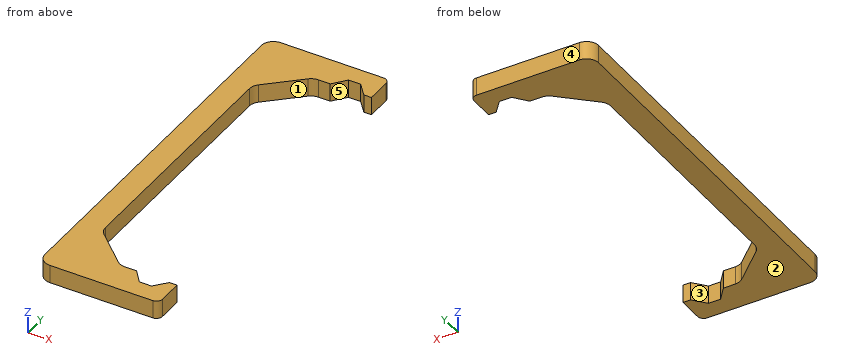
```python
from build123d import *

# Parameters (mm, degrees)
F1_DEPTH = 9.525


with BuildPart() as f1:
    # F0 (on Top) → F1 (new body)
    with BuildSketch(Plane.XY):
        with BuildLine():
            Line((-2.285999, 147.979229), (-46.735999, 147.979229))
            ThreePointArc((-46.735999, 147.979229), (-51.226127, 146.119357), (-53.085999, 141.629229))
            Line((-53.085999, 141.629229), (-53.085999, -48.870771))
            ThreePointArc((-53.085999, -48.870771), (-51.226127, -53.360899), (-46.735999, -55.220771))
            Line((-46.735999, -55.220771), (-2.285999, -55.220771))
            Line((-2.285999, -55.220771), (7.239001, -55.220771))
            ThreePointArc((7.239001, -55.220771), (9.484065, -54.290835), (10.414001, -52.045771))
            Line((10.414001, -52.045771), (10.414001, -39.218631))
            Line((10.414001, -39.218631), (6.426201, -39.218631))
            Line((6.426201, -39.218631), (0.889001, -45.695771))
            Line((0.889001, -45.695771), (-5.460999, -45.695771))
            Line((-5.460999, -45.695771), (-10.998199, -38.880926))
            Line((-10.998199, -38.880926), (-17.265751, -38.880926))
            ThreePointArc((-17.265751, -38.880926), (-19.578043, -38.444961), (-21.57283, -37.196928))
            Line((-21.57283, -37.196928), (-38.343077, -21.7167))
            ThreePointArc((-38.343077, -21.7167), (-39.85289, -19.597514), (-40.385999, -17.050698))
            Line((-40.385999, -17.050698), (-40.385999, 109.809156))
            ThreePointArc((-40.385999, 109.809156), (-39.85289, 112.355972), (-38.343077, 114.475157))
            Line((-38.343077, 114.475157), (-21.57283, 129.955386))
            ThreePointArc((-21.57283, 129.955386), (-19.578043, 131.203419), (-17.265751, 131.639384))
            Line((-17.265751, 131.639384), (-10.998199, 131.639384))
            Line((-10.998199, 131.639384), (-5.460999, 138.454229))
            Line((-5.460999, 138.454229), (0.889001, 138.454229))
            Line((0.889001, 138.454229), (6.426201, 131.977089))
            Line((6.426201, 131.977089), (10.414001, 131.977089))
            Line((10.414001, 131.977089), (10.414001, 144.804229))
            ThreePointArc((10.414001, 144.804229), (9.484065, 147.049293), (7.239001, 147.979229))
            Line((7.239001, 147.979229), (-2.285999, 147.979229))
        make_face()
    extrude(amount=F1_DEPTH)


solid = f1.part
```
Source: CAD feature listing. Evaluate the final solid. Frame: model axes, mm. Face numbers are marked on the shaded views. A direction names the side the tool comes from. Give positions to 0.01 mm unless a question says otherwise; leave off trailing zeros. Write each loop counter-clockwise with the first axis right and the second up, starting at its lowest first coordinate (ties: lowest second). Pieces come first, ordered by that corner, then holes.
1. Section query D-D (y = 52). Return the cut outline in (x, z) (3 decimals), then the cut area to 3 significant figures.
2. Access query for the marked faces 4 and 5. Directions: +Z, -Z, +X, -X, +Y, -Y. A direction counts if a zero-diameter tool reaches every point of the face in a straight line with its end or side. Return the directions, or none.
3. Section query A-A (y = -41). Return the cut outline in (x, z) (3 decimals), then the cut area to 3 significant figures.
4. Section query B-B (x = -31). Return the cut outline in (y, z) (3 decimals), then the cut area to 3 significant figures.
5. Material intervals for line 1 along Y through (x, z) = (-2, 2.75); line 2 along Y through (x, z) = (-16, 6.5); line 3 along X through (y, z) = (-15, 2.5), sorted ascending.
6. Section query C-C (z = 1.5). Return the cut outline in (x, y) (3 decimals), then the cut area to 3 significant figures.
7. Pull-direction query (X, two-part tool) for the marked faces 1, 2 and 3; classes: +X half, -X half, draft (parallel to the pull), parting line (faces both ways), or undercut.
8. First-contact query: pin 1 (1.2 mm diameter, centred on x = 9, z = 4.5, fed in from -Y); pin 2 (3 mm diameter, centred on y = 21.5, z = 8.5, fed in from +X). Flat tips, straight axial feed; report the tip coordinate or a pass-through.
Output values:
1. outline: (-53.086, 0) - (-40.386, 0) - (-40.386, 9.525) - (-53.086, 9.525) - close
1. area: 121 mm2
2. face 4: +Z, -Z, +X, -X, +Y
2. face 5: +Z, -Z
3. outline: (-53.086, 0) - (-9.276, 0) - (-9.276, 9.525) - (-53.086, 9.525) - close; (4.903, 0) - (10.414, 0) - (10.414, 9.525) - (4.903, 9.525) - close
3. area: 470 mm2
4. outline: (-55.221, 0) - (-28.495, 0) - (-28.495, 9.525) - (-55.221, 9.525) - close; (121.253, 0) - (147.979, 0) - (147.979, 9.525) - (121.253, 9.525) - close
4. area: 509 mm2
5. line 1: y = -55.22 to -45.7, 138.45 to 147.98
5. line 2: y = -55.22 to -38.88, 131.64 to 147.98
5. line 3: x = -53.09 to -40.39
6. outline: (-53.086, -48.871) arc R6.35 ccw to (-46.736, -55.221) - (7.239, -55.221) arc R3.175 ccw to (10.414, -52.046) - (10.414, -39.219) - (6.426, -39.219) - (0.889, -45.696) - (-5.461, -45.696) - (-10.998, -38.881) - (-17.266, -38.881) arc R6.35 cw to (-21.573, -37.197) - (-38.343, -21.717) arc R6.35 cw to (-40.386, -17.051) - (-40.386, 109.809) arc R6.35 cw to (-38.343, 114.475) - (-21.573, 129.955) arc R6.35 cw to (-17.266, 131.639) - (-10.998, 131.639) - (-5.461, 138.454) - (0.889, 138.454) - (6.426, 131.977) - (10.414, 131.977) - (10.414, 144.804) arc R3.175 ccw to (7.239, 147.979) - (-46.736, 147.979) arc R6.35 ccw to (-53.086, 141.629) - close
6. area: 4,450 mm2
7. face 1: +X half
7. face 2: draft
7. face 3: undercut
8. pin 1: stops at y = -55
8. pin 2: stops at x = -40.39
